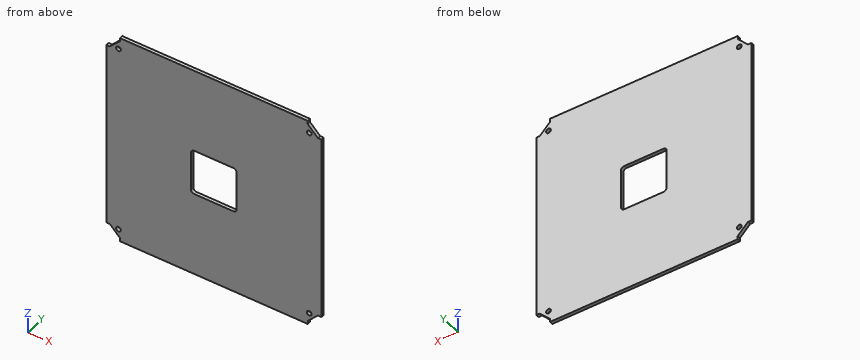
from build123d import *

# Parameters (mm, degrees)
BOSS_EXTRUDE1_DEPTH = 3.175
CUT_EXTRUDE1_REACH  = 5.175
SKETCH3_R           = 2.286
CUT_EXTRUDE2_REACH  = 5.175
SKETCH5_W           = 44.45
SKETCH5_H           = 44.45
FILLET1_R           = 3.175


with BuildPart() as part:
    # Sketch1 → Boss-Extrude1 (new body)
    with BuildSketch(Plane(origin=(0, 0, 0), x_dir=(1, 0, 0), z_dir=(0, 1, 0))):
        Polygon((-91.233267746, 104.4575), (-91.233267746, 101.1555), (-101.1555, 91.321365209), (-104.4575, 91.321365209), (-104.4575, -91.233267746), (-101.1555, -91.233267746), (-91.321365209, -101.1555), (-91.321365209, -104.4575), (91.233267746, -104.4575), (91.233267746, -101.1555), (101.1555, -91.321365209), (104.4575, -91.321365209), (104.4575, 91.233267746), (101.1555, 91.233267746), (91.321365209, 101.1555), (91.321365209, 104.4575), align=None)
    extrude(amount=BOSS_EXTRUDE1_DEPTH)

    # Sketch3 → Cut-Extrude1 (cut, up to next)
    with BuildSketch(Plane(origin=(0, 3.175, 0), x_dir=(1, 0, 0), z_dir=(0, 1, 0)), mode=Mode.PRIVATE) as cut_extrude1_sk1:
        with Locations((-92.73413, 92.73413)):
            Circle(SKETCH3_R)
    cut_extrude1_tool1 = extrude(cut_extrude1_sk1.sketch, amount=-CUT_EXTRUDE1_REACH, mode=Mode.PRIVATE) & part.part
    add(cut_extrude1_tool1.solids().sort_by_distance((-92.73413, 3.175, -92.73413))[0], mode=Mode.SUBTRACT)
    # Sketch3 → Cut-Extrude1 (cut, up to next)
    with BuildSketch(Plane(origin=(0, 3.175, 0), x_dir=(1, 0, 0), z_dir=(0, 1, 0)), mode=Mode.PRIVATE) as cut_extrude1_sk2:
        with Locations((92.73413, 92.73413)):
            Circle(SKETCH3_R)
    cut_extrude1_tool2 = extrude(cut_extrude1_sk2.sketch, amount=-CUT_EXTRUDE1_REACH, mode=Mode.PRIVATE) & part.part
    add(cut_extrude1_tool2.solids().sort_by_distance((92.73413, 3.175, -92.73413))[0], mode=Mode.SUBTRACT)
    # Sketch3 → Cut-Extrude1 (cut, up to next)
    with BuildSketch(Plane(origin=(0, 3.175, 0), x_dir=(1, 0, 0), z_dir=(0, 1, 0)), mode=Mode.PRIVATE) as cut_extrude1_sk3:
        with Locations((92.73413, -92.73413)):
            Circle(SKETCH3_R)
    cut_extrude1_tool3 = extrude(cut_extrude1_sk3.sketch, amount=-CUT_EXTRUDE1_REACH, mode=Mode.PRIVATE) & part.part
    add(cut_extrude1_tool3.solids().sort_by_distance((92.73413, 3.175, 92.73413))[0], mode=Mode.SUBTRACT)
    # Sketch3 → Cut-Extrude1 (cut, up to next)
    with BuildSketch(Plane(origin=(0, 3.175, 0), x_dir=(1, 0, 0), z_dir=(0, 1, 0)), mode=Mode.PRIVATE) as cut_extrude1_sk4:
        with Locations((-92.73413, -92.73413)):
            Circle(SKETCH3_R)
    cut_extrude1_tool4 = extrude(cut_extrude1_sk4.sketch, amount=-CUT_EXTRUDE1_REACH, mode=Mode.PRIVATE) & part.part
    add(cut_extrude1_tool4.solids().sort_by_distance((-92.73413, 3.175, 92.73413))[0], mode=Mode.SUBTRACT)

    # Sketch5 → Cut-Extrude2 (cut, up to next)
    with BuildSketch(Plane(origin=(0, 3.175, 0), x_dir=(1, 0, 0), z_dir=(0, 1, 0)), mode=Mode.PRIVATE) as cut_extrude2_sk1:
        Rectangle(SKETCH5_W, SKETCH5_H)
    cut_extrude2_tool1 = extrude(cut_extrude2_sk1.sketch, amount=-CUT_EXTRUDE2_REACH, mode=Mode.PRIVATE) & part.part
    add(cut_extrude2_tool1.solids().sort_by_distance((0, 3.175, 0))[0], mode=Mode.SUBTRACT)

    # Fillet1
    fillet1_edges = [part.edges().sort_by_distance(p)[0] for p in [
        (-22.225, 1.5875, 22.225),
        (-22.225, 1.5875, -22.225),
        (22.225, 1.5875, -22.225),
        (22.225, 1.5875, 22.225),
    ]]
    fillet(fillet1_edges, radius=FILLET1_R)


solid = part.part
The model under review builds one solid part; all positions refer to its coordinate system, in mm. Round coordinates to 2 decimals unless told otherwise and drop trailing zeros. Loops run counter-clockwise (first coordinate to the right, second up) from the corner with the lowest first, then second, coordinate; pieces in that order, holes last. Notation, with made-up numbers: (-6, -7) -> (3, -7) arc R21 ccw to (3, 14) -> close; hole circle Ø9 at (79.25, -28.75). An arc over 180 degrees is marked (long way). Write item = value, one per line. Start each with the question number.
Item 1: Take a section at B-B on z = 15. Give the boundary of the cut face in (x, y) (1 decimal), plus the area to 3 significant figures.
Item 2: Insertion check: pin 1 (4 mm diameter, centred on x = 92.73, z = 92.73, fed in from +Y); pin 2 (1 mm diameter, centred on y = 1, z = -102.5, fed in from +X); pin 3 (6 mm diameter, centred on x = -3.5, z = -75.5, fed in from -Y); pin 4 (1 mm diameter, centred on x = 103, y = 2, fed in from -Z). Each pin has a flat end and moves straight along its axis. Give the tip position at first contact, or say it passes through.
Item 3: Take a section at A-A on x = -13.5. Give the boundary of the cut face in (y, z) (1 decimal), plus the area to 3 significant figures.
Item 4: Take a section at C-C on y = 1.6. Count the separate pieces of the cut face and the enclosed holes in it, plus the area to 3 significant figures.
Item 5: To check wall thickness, follow L1, parallel to Z at x = 1, y = 1.8 (1 decimal); L2, parallel to Z at x = -20, y = 2.6. State the ranges of each line that lie inside material, in increasing order.
Result:
q1.outline = (-104.5, 0) -> (-22.2, 0) -> (-22.2, 3.2) -> (-104.5, 3.2) -> close; (22.2, 0) -> (104.5, 0) -> (104.5, 3.2) -> (22.2, 3.2) -> close
q1.area = 522 mm²
q2.pin_1 = through
q2.pin_2 = 91.32
q2.pin_3 = 0
q2.pin_4 = -91.23
q3.outline = (0, -104.5) -> (3.2, -104.5) -> (3.2, -22.2) -> (0, -22.2) -> close; (0, 22.2) -> (3.2, 22.2) -> (3.2, 104.5) -> (0, 104.5) -> close
q3.area = 522 mm²
q4.separate_pieces = 1
q4.enclosed_holes = 5
q4.area = 41,100 mm²
q5.L1 = -104.5 to -22.2, 22.2 to 104.5
q5.L2 = -104.46 to -22.08, 22.08 to 104.46
